from build123d import *

# Parameters (mm, degrees)
EXTRUDE_2549_DEPTH  = 10
SKETCH_9_R          = 10
EXTRUDE_3976_DEPTH  = 29
EXTRUDE_1_DEPTH     = 19.5
CUT_EXTRUDE_1_DEPTH = 5


with BuildPart() as part:
    # Sketch 8 → Extrude 2549 (new body)
    with BuildSketch(Plane.XY):
        with BuildLine():
            ThreePointArc((14.816916277, 45.813551402), (18.814169361, 44.322111088), (22.663708414, 42.482688485))
            ThreePointArc((22.663708414, 42.482688485), (29.561909195, 46.788200222), (37.378099503, 44.545484367))
            ThreePointArc((37.378099503, 44.545484367), (25.54998575, 52.236201318), (12.217842113, 56.851973001))
            ThreePointArc((12.217842113, 56.851973001), (14.287540581, 52.717951856), (15, 48.15))
            ThreePointArc((15, 48.15), (14.954159023, 46.978194587), (14.816916277, 45.813551402))
        make_face()
        with BuildLine():
            ThreePointArc((14.816916277, 45.813551402), (13.130097556, 40.897377152), (9.866842754, 36.851973001))
            ThreePointArc((9.866842754, 36.851973001), (17.612447876, 33.84116103), (24.52234731, 29.224595505))
            ThreePointArc((24.52234731, 29.224595505), (21.04706312, 35.496725725), (22.663708414, 42.482688485))
            ThreePointArc((22.663708414, 42.482688485), (18.814169361, 44.322111088), (14.816916277, 45.813551402))
        make_face()
        with BuildLine():
            ThreePointArc((-9.278843612, 59.935714286), (-13.964608204, 53.626286855), (-14.816916277, 45.813551402))
            ThreePointArc((-14.816916277, 45.813551402), (-9.469116127, 47.209727173), (-3.996547888, 47.983852544))
            ThreePointArc((-3.996547888, 47.983852544), (-0.083091657, 52.149136879), (4, 48.15))
            ThreePointArc((4, 48.15), (3.999136879, 48.066908343), (3.996547888, 47.983852544))
            ThreePointArc((3.996547888, 47.983852544), (9.469116127, 47.209727173), (14.816916277, 45.813551402))
            ThreePointArc((14.816916277, 45.813551402), (14.954159023, 46.978194587), (15, 48.15))
            ThreePointArc((15, 48.15), (14.287540581, 52.717951856), (12.217842113, 56.851973001))
            ThreePointArc((12.217842113, 56.851973001), (6.143300009, 57.824582705), (0, 58.15))
            ThreePointArc((0, 58.15), (-4.724555913, 58.600487348), (-9.278843612, 59.935714286))
        make_face()
        with BuildLine():
            ThreePointArc((-3.996547888, 47.983852544), (-9.469116127, 47.209727173), (-14.816916277, 45.813551402))
            ThreePointArc((-14.816916277, 45.813551402), (-14.247332672, 43.458144105), (-13.305901978, 41.225191516))
            ThreePointArc((-13.305901978, 41.225191516), (-6.828320261, 38.928798681), (0, 38.15))
            ThreePointArc((0, 38.15), (4.975928557, 37.824101245), (9.866842754, 36.851973001))
            ThreePointArc((9.866842754, 36.851973001), (13.130097556, 40.897377152), (14.816916277, 45.813551402))
            ThreePointArc((14.816916277, 45.813551402), (9.469116127, 47.209727173), (3.996547888, 47.983852544))
            ThreePointArc((3.996547888, 47.983852544), (0, 44.15), (-3.996547888, 47.983852544))
        make_face()
        with BuildLine():
            ThreePointArc((-14.816916277, 45.813551402), (-16.67536312, 45.170286304), (-18.505991963, 44.451667702))
            ThreePointArc((-18.505991963, 44.451667702), (-15.987547848, 42.706914024), (-13.305901978, 41.225191516))
            ThreePointArc((-13.305901978, 41.225191516), (-14.247332672, 43.458144105), (-14.816916277, 45.813551402))
        make_face()
        with BuildLine():
            ThreePointArc((-20.602788665, 68.989311485), (-25.448248321, 67.352703416), (-30.165303473, 65.376253077))
            ThreePointArc((-30.165303473, 65.376253077), (-26.489305732, 53.713928503), (-18.505991963, 44.451667702))
            ThreePointArc((-18.505991963, 44.451667702), (-16.67536312, 45.170286304), (-14.816916277, 45.813551402))
            ThreePointArc((-14.816916277, 45.813551402), (-13.964608204, 53.626286855), (-9.278843612, 59.935714286))
            ThreePointArc((-9.278843612, 59.935714286), (-15.611530753, 63.62360485), (-20.602788665, 68.989311485))
        make_face()
        with BuildLine():
            ThreePointArc((-8.237889177, 60.685437045), (-8.766384828, 60.32170888), (-9.278843612, 59.935714286))
            ThreePointArc((-9.278843612, 59.935714286), (-4.724555913, 58.600487348), (0, 58.15))
            ThreePointArc((0, 58.15), (-4.309618866, 58.798198675), (-8.237889177, 60.685437045))
        make_face()
        with BuildLine():
            ThreePointArc((-14.473600663, 70.530240917), (-17.555110024, 69.827058595), (-20.602788665, 68.989311485))
            ThreePointArc((-20.602788665, 68.989311485), (-15.611530753, 63.62360485), (-9.278843612, 59.935714286))
            ThreePointArc((-9.278843612, 59.935714286), (-8.766384828, 60.32170888), (-8.237889177, 60.685437045))
            ThreePointArc((-8.237889177, 60.685437045), (-12.376711337, 64.961157534), (-14.473600663, 70.530240917))
        make_face()
    extrude(amount=EXTRUDE_2549_DEPTH)

    # Sketch 9 → Extrude 3976 (add)
    with BuildSketch(Plane.XY):
        with Locations(Location((30.950223406, 36.885039936, 0), (0, 0, 230))):
            Circle(SKETCH_9_R)
    extrude(amount=EXTRUDE_3976_DEPTH)

    # Sketch 11 → Extrude 1 (add)
    with BuildSketch(Plane.XY):
        with BuildLine():
            ThreePointArc((-30.323937444, 68.473937444), (-30.284252984, 66.923065659), (-30.165303473, 65.376253077))
            ThreePointArc((-30.165303473, 65.376253077), (-25.448248321, 67.352703416), (-20.602788665, 68.989311485))
            ThreePointArc((-20.602788665, 68.989311485), (-23.875402789, 75.736152033), (-25, 83.15))
            Line((-25, 83.15), (-25, 99.176328781))
            Line((-25, 99.176328781), (-30.323937444, 99.176328781))
            Line((-30.323937444, 99.176328781), (-30.323937444, 92.15))
            Line((-30.323937444, 92.15), (-26.682795781, 92.15))
            Line((-26.682795781, 92.15), (-26.682795781, 86.338672823))
            Line((-26.682795781, 86.338672823), (-30.323937444, 86.338672823))
            Line((-30.323937444, 86.338672823), (-30.323937444, 68.473937444))
        make_face()
        with BuildLine():
            ThreePointArc((-25, 83.15), (-23.875402789, 75.736152033), (-20.602788665, 68.989311485))
            ThreePointArc((-20.602788665, 68.989311485), (-17.555110024, 69.827058595), (-14.473600663, 70.530240917))
            ThreePointArc((-14.473600663, 70.530240917), (-14.606270011, 71.661967819), (-14.650582479, 72.800582479))
            Line((-14.650582479, 72.800582479), (-14.650582479, 99.176328781))
            Line((-14.650582479, 99.176328781), (-25, 99.176328781))
            Line((-25, 99.176328781), (-25, 83.15))
        make_face()
    extrude(amount=EXTRUDE_1_DEPTH)

    # Sketch 12 → Cut-Extrude 1 (cut)
    with BuildSketch(Plane.XY):
        with BuildLine():
            ThreePointArc((-25, 83.15), (-23.875402789, 75.736152033), (-20.602788665, 68.989311485))
            ThreePointArc((-20.602788665, 68.989311485), (-17.555110024, 69.827058595), (-14.473600663, 70.530240917))
            ThreePointArc((-14.473600663, 70.530240917), (-14.606270011, 71.661967819), (-14.650582479, 72.800582479))
            Line((-14.650582479, 72.800582479), (-14.650582479, 99.176328781))
            Line((-14.650582479, 99.176328781), (-25, 99.176328781))
            Line((-25, 99.176328781), (-25, 83.15))
        make_face()
        with BuildLine():
            ThreePointArc((-30.323937444, 68.473937444), (-30.284252984, 66.923065659), (-30.165303473, 65.376253077))
            ThreePointArc((-30.165303473, 65.376253077), (-25.448248321, 67.352703416), (-20.602788665, 68.989311485))
            ThreePointArc((-20.602788665, 68.989311485), (-23.875402789, 75.736152033), (-25, 83.15))
            Line((-25, 83.15), (-25, 99.176328781))
            Line((-25, 99.176328781), (-30.323937444, 99.176328781))
            Line((-30.323937444, 99.176328781), (-30.323937444, 92.15))
            Line((-30.323937444, 92.15), (-26.682795781, 92.15))
            Line((-26.682795781, 92.15), (-26.682795781, 86.338672823))
            Line((-26.682795781, 86.338672823), (-30.323937444, 86.338672823))
            Line((-30.323937444, 86.338672823), (-30.323937444, 68.473937444))
        make_face()
    extrude(amount=CUT_EXTRUDE_1_DEPTH, mode=Mode.SUBTRACT)


solid = part.part
Can you work these out from the model? Positions are in its coordinate system, mm. A direction names the side the tool comes from. Round coordinates to 2 decimals unless told otherwise and drop trailing zeros. Order: outer loops, then holes, each group sorted by start corner. A loop starts at its lowest first (then second) coordinate and runs counter-clockwise, first axis right, second up. Notation, with made-up numbers: (-33, 17) -> (-24, 17) arc R32 ccw to (-24, 53) -> close; hole circle Ø5 at (-9, 1.5). An arc over 180 degrees is marked (long way). Write each question's results on one line, items separated by ' | '. Start each with the question number.
Item 1: Will these pins go through, and if not, where does the flat tip stop? pin 1 (5 mm diameter, centred on x = -18.5, y = 78, fed in from +Z); pin 2 (5 mm diameter, centred on x = 1, z = 11, fed in from +Y); pin 3 (3 mm diameter, centred on y = 90, z = 12.5, fed in from -X); pin 4 (2 mm diameter, centred on x = 18, y = 53, fed in from -Z).
Item 2: If we section it at B-B, the plane x = 33: Write out the boundary of the cut face in (y, z), then the cut area to 3 significant figures.
Item 3: Which directions (+Z, -Z, +X, -X, +Y, -Y) give clear straight access to the entire face, cutting with the end or side of a thin tool? Please do faces 1 (the flat face through (-29, 92.15, 12)), 2 (the flat face through (-30.324, 96, 12)).
Item 4: Thinking about a two-plate mould opening in Y: for faces 3 (the flat face through (-14.651, 86, 12)), 4 (the flat face through (-28, 86.339, 12)), 5 (the cylindrical face through (39.382, 31.509, 17.519)), which applies, +Y half, -Y half, draft (parallel to the pull), parting line (faces both ways), or undercut?
Item 5: If we section it at A-A, the plane z = 18: Write out the boundary of the cut face in (x, y).
Item 6: Please list where these lines run through material, in increasing order: L1, parallel to X at y = 94.5, z = 8; L2, parallel to Z at x = -21.5, y = 77.5; L3, parallel to Y at x = -22.5, z = 8.5.
Item 7: If we section it at C-C, the plane y = 71.5: Write out the boundary of the cut face in (x, z), then the cut area to 3 significant figures.
Results:
1) pin 1: stops at z = 19.5 | pin 2: stops at y = 58.21 | pin 3: stops at x = -26.68 | pin 4: stops at z = 0
2) outline: (27.1, 0) -> (47.88, 0) -> (47.88, 10) -> (46.67, 10) -> (46.67, 29) -> (27.1, 29) -> close | area: 580 mm2
3) face 1: +Z, -Z, -X | face 2: +Z, -Z, -X, +Y, -Y
4) face 3: draft | face 4: undercut | face 5: parting line
5) outline: (-30.32, 68.47) arc R30.32 ccw to (-30.17, 65.38) arc R72 cw to (-14.47, 70.53) arc R14.65 cw to (-14.65, 72.8) -> (-14.65, 99.18) -> (-30.32, 99.18) -> (-30.32, 92.15) -> (-26.68, 92.15) -> (-26.68, 86.34) -> (-30.32, 86.34) -> close; circle Ø20 at (30.95, 36.89)
6) L1: x = -30.32 to -14.65 | L2: z = 5 to 19.5 | L3: y = 48.14 to 99.18
7) outline: (-30.32, 5) -> (-14.59, 5) -> (-14.59, 19.5) -> (-30.32, 19.5) -> close | area: 228 mm2
